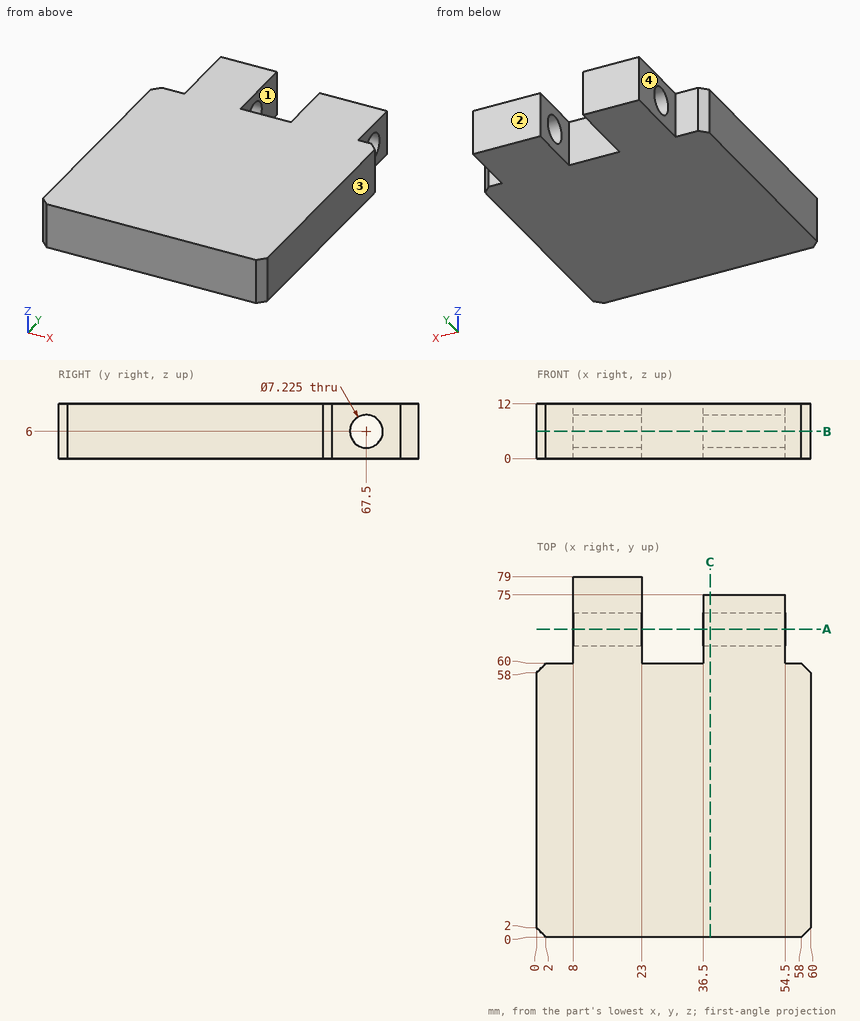
Answer from the drawing. Dimensions are ordinates in mm from the lowest x, y and z of the part. A direction names the side the tool comes from. Coordinates: 2 decimals unless noted, no trailing zeros. Write each loop counter-clockwise with the first axis right and the second up, starting at its lowest first coordinate (ties: lowest second). Pieces come first, ordered by that corner, then holes. Notation, with made-up numbers: (-36.5, 87.5) - (-25.5, 87.5) arc R17 ccw to (-25.5, 95.5) - close; hole circle Ø2 at (-9, 4.25). An arc over 180 degrees is marked (long way). Answer as CSV lines item,"result".
1. A tool of negligible diameter and unlimited length cuts with its end or side. For the marked faces 1, 2, 3 and 4, from which of +Z, -Z, +X, -X, +Y, -Y can it reach the whole face along a straight path? Write none if from no direction.
Computed values:
face 1,"+Z, -Z, +Y"
face 2,"+Z, -Z, +X, +Y"
face 3,"+Z, -Z, +X, +Y, -Y"
face 4,"+Z, -Z, -X, +Y"
2. Find section B-B (z = 6). Give the vertices of the cut face in (x, y), plus the area to 3 significant figures.
Computed values:
outline,"(0, 2) - (2, 0) - (58, 0) - (60, 2) - (60, 58) - (58, 60) - (54.5, 60) - (54.5, 63.89) - (36.5, 63.89) - (36.5, 60) - (23, 60) - (23, 63.89) - (8, 63.89) - (8, 60) - (2, 60) - (0, 58) - close; (8, 71.11) - (23, 71.11) - (23, 79) - (8, 79) - close; (36.5, 71.11) - (54.5, 71.11) - (54.5, 75) - (36.5, 75) - close"
area,"3,910 mm²"
3. Find section A-A (y = 67.5). Give the vertices of the cut face in (x, z).
Computed values:
outline,"(8, 0) - (23, 0) - (23, 2.39) - (8, 2.39) - close; (8, 9.61) - (23, 9.61) - (23, 12) - (8, 12) - close; (36.5, 0) - (54.5, 0) - (54.5, 2.39) - (36.5, 2.39) - close; (36.5, 9.61) - (54.5, 9.61) - (54.5, 12) - (36.5, 12) - close"
4. Given P1, Ø3.5, axis at x = 42.5, z = 3.5, coming from the +Y side; P2, Ø1, axis at x = 19, y = 10.5, coming from the -Z side; P3, Ø1.8, axis at x = 56, z = 6, coming from the +Y side; P4, Ø6, axis at y = 71, z = 8.5, coming from the -X side, each flat-ended and moving along its own axis, determine where each tip first touches the part or whether it passes through.
Computed values:
P1,"stops at y = 75"
P2,"stops at z = 0"
P3,"stops at y = 60"
P4,"stops at x = 8"
5. Find section C-C (x = 38). Give the vertices of the cut face in (y, z) (1 decimal).
Computed values:
outline,"(0, 0) - (75, 0) - (75, 12) - (0, 12) - close; hole circle Ø7.2 at (67.5, 6)"
6. Straight lines are drawn through the part: line 1 (X direction, y = 74.5, z = 0.5); line 2 (Y direction, x = 42.25, z = 6); line 3 (Y direction, x = 12, z = 6). For each, find the intervals that lie inside material, in ascending order. Write a range as [from, to].
Computed values:
line 1,"x = [8, 23], [36.5, 54.5]"
line 2,"y = [0, 63.89], [71.11, 75]"
line 3,"y = [0, 63.89], [71.11, 79]"
